```python
from build123d import *

# Parameters (mm, degrees)
SKETCH1_W           = 282
SKETCH1_H           = 170
BOSS_EXTRUDE1_DEPTH = 60
CUT_EXTRUDE4_DEPTH  = 5
SKETCH8_W           = 160
SKETCH8_H           = 50
CUT_EXTRUDE5_DEPTH  = 279
CUT_EXTRUDE6_DEPTH  = 5
SKETCH10_R          = 5
CUT_EXTRUDE7_DEPTH  = 5
CUT_EXTRUDE8_DEPTH  = 5
CUT_EXTRUDE9_START  = -5
CUT_EXTRUDE9_DEPTH  = 5
SKETCH14_W          = 185
SKETCH14_H          = 5
BOSS_EXTRUDE2_DEPTH = 10
SKETCH15_W          = 185
SKETCH15_H          = 5
BOSS_EXTRUDE3_DEPTH = 10
SKETCH16_W          = 97
SKETCH16_H          = 15
CUT_EXTRUDE10_DEPTH = 170
BOSS_EXTRUDE4_DEPTH = 160
SKETCH18_W          = 15
SKETCH18_H          = 10
CUT_EXTRUDE11_DEPTH = 340.888216918


with BuildPart() as part:
    # Sketch1 → Boss-Extrude1 (new body)
    with BuildSketch(Plane(origin=(0, 0, 0), x_dir=(1, 0, 0), z_dir=(0, 1, 0))):
        with Locations((141, 85)):
            Rectangle(SKETCH1_W, SKETCH1_H)
    extrude(amount=BOSS_EXTRUDE1_DEPTH)

    # Sketch7 → Cut-Extrude4 (cut)
    with BuildSketch(Plane.XZ):
        with BuildLine():
            Line((13.5, -37.5), (13.5, -132.5))
            ThreePointArc((13.5, -132.5), (11, -135), (8.5, -132.5))
            Line((8.5, -132.5), (8.5, -37.5))
            ThreePointArc((8.5, -37.5), (11, -35), (13.5, -37.5))
        make_face()
        with BuildLine():
            Line((58.5, -37.5), (58.5, -132.5))
            ThreePointArc((58.5, -132.5), (56, -135), (53.5, -132.5))
            Line((53.5, -132.5), (53.5, -37.5))
            ThreePointArc((53.5, -37.5), (56, -35), (58.5, -37.5))
        make_face()
        with BuildLine():
            Line((28.5, -37.5), (28.5, -132.5))
            ThreePointArc((28.5, -132.5), (26, -135), (23.5, -132.5))
            Line((23.5, -132.5), (23.5, -37.5))
            ThreePointArc((23.5, -37.5), (26, -35), (28.5, -37.5))
        make_face()
        with BuildLine():
            Line((43.5, -37.5), (43.5, -132.5))
            ThreePointArc((43.5, -132.5), (41, -135), (38.5, -132.5))
            Line((38.5, -132.5), (38.5, -37.5))
            ThreePointArc((38.5, -37.5), (41, -35), (43.5, -37.5))
        make_face()
    extrude(amount=-CUT_EXTRUDE4_DEPTH, mode=Mode.SUBTRACT)

    # Sketch8 → Cut-Extrude5 (cut)
    with BuildSketch(Plane(origin=(282, 0, 0), x_dir=(0, 0, -1), z_dir=(1, 0, 0))):
        with Locations((85, 30)):
            Rectangle(SKETCH8_W, SKETCH8_H)
    extrude(amount=-CUT_EXTRUDE5_DEPTH, mode=Mode.SUBTRACT)

    # Sketch9 → Cut-Extrude6 (cut)
    with BuildSketch(Plane.XY):
        Polygon((217.15, 25.8), (227.05, 25.8), (227.05, 8.15), (224.8, 5), (219.4, 5), (217.15, 8.15), align=None)
        Polygon((162.25, 25.8), (172.15, 25.8), (172.15, 8.15), (169.9, 5), (164.5, 5), (162.25, 8.15), align=None)
    extrude(amount=-CUT_EXTRUDE6_DEPTH, mode=Mode.SUBTRACT)

    # Sketch10 → Cut-Extrude7 (cut)
    with BuildSketch(Plane.ZY):
        with Locations((-129.202249563, 20)):
            Circle(SKETCH10_R)
        with Locations((-114.202249563, 20)):
            Circle(SKETCH10_R)
        with Locations((-99.202249563, 20)):
            Circle(SKETCH10_R)
        with Locations((-43.390057257, 20)):
            Circle(SKETCH10_R)
        with Locations((-58.390057257, 20)):
            Circle(SKETCH10_R)
        with Locations((-73.390057257, 20)):
            Circle(SKETCH10_R)
    extrude(amount=-CUT_EXTRUDE7_DEPTH, mode=Mode.SUBTRACT)

    # Sketch11 → Cut-Extrude8 (cut)
    with BuildSketch(Plane.XY):
        with BuildLine():
            Line((11, 13.5), (56, 13.5))
            ThreePointArc((56, 13.5), (58.5, 11), (56, 8.5))
            Line((56, 8.5), (11, 8.5))
            ThreePointArc((11, 8.5), (8.5, 11), (11, 13.5))
        make_face()
        with BuildLine():
            Line((11, 23.5), (56, 23.5))
            ThreePointArc((56, 23.5), (58.5, 21), (56, 18.5))
            Line((56, 18.5), (11, 18.5))
            ThreePointArc((11, 18.5), (8.5, 21), (11, 23.5))
        make_face()
    extrude(amount=-CUT_EXTRUDE8_DEPTH, mode=Mode.SUBTRACT)

    # Sketch12 → Cut-Extrude9 (cut)
    with BuildSketch(Plane(origin=(0, 0, -170), x_dir=(-1, 0, 0), z_dir=(0, 0, -1)).offset(CUT_EXTRUDE9_START)):
        with BuildLine():
            Line((-56, 13.5), (-11, 13.5))
            ThreePointArc((-11, 13.5), (-8.5, 11), (-11, 8.5))
            Line((-11, 8.5), (-56, 8.5))
            ThreePointArc((-56, 8.5), (-58.5, 11), (-56, 13.5))
        make_face()
        with BuildLine():
            Line((-56, 23.5), (-11, 23.5))
            ThreePointArc((-11, 23.5), (-8.5, 21), (-11, 18.5))
            Line((-11, 18.5), (-56, 18.5))
            ThreePointArc((-56, 18.5), (-58.5, 21), (-56, 23.5))
        make_face()
    extrude(amount=CUT_EXTRUDE9_DEPTH, mode=Mode.SUBTRACT)

    # Sketch14 → Boss-Extrude2 (add)
    with BuildSketch(Plane.XY):
        with Locations((189.5, 57.5)):
            Rectangle(SKETCH14_W, SKETCH14_H)
    extrude(amount=BOSS_EXTRUDE2_DEPTH)

    # Sketch15 → Boss-Extrude3 (add)
    with BuildSketch(Plane(origin=(0, 0, -170), x_dir=(-1, 0, 0), z_dir=(0, 0, -1))):
        with Locations((-189.5, 57.5)):
            Rectangle(SKETCH15_W, SKETCH15_H)
    extrude(amount=BOSS_EXTRUDE3_DEPTH)

    # Sketch16 → Cut-Extrude10 (cut)
    with BuildSketch(Plane.XY):
        with Locations((48.5, 52.5)):
            Rectangle(SKETCH16_W, SKETCH16_H)
    extrude(amount=-CUT_EXTRUDE10_DEPTH, mode=Mode.SUBTRACT)

    # Sketch17 → Boss-Extrude4 (add)
    with BuildSketch(Plane.XY.offset(-165)):
        Polygon((3, 45), (97, 45), (97, 55), (102, 55), (102, 40), (3, 40), align=None)
    extrude(amount=BOSS_EXTRUDE4_DEPTH)

    # Sketch18 → Cut-Extrude11 (cut, through all)
    with BuildSketch(Plane.XY):
        with Locations((69.5, 22)):
            Rectangle(SKETCH18_W, SKETCH18_H)
    extrude(amount=-CUT_EXTRUDE11_DEPTH, mode=Mode.SUBTRACT)


solid = part.part
```
The listing builds one solid part. Answer for the finished solid, in the listing's coordinates (mm). A direction names the side the tool comes from. Give positions to 0.01 mm unless a question says otherwise; leave off trailing zeros. Order: outer loops, then holes, each group sorted by start corner. A loop starts at its lowest first (then second) coordinate and runs counter-clockwise, first axis right, second up.
1) Given P1, Ø5, axis at x = 147, y = 50.5, coming from the -Z side; P2, Ø8, axis at y = 9.5, z = -30, coming from the -X side; P3, Ø5, axis at y = 11.5, z = -103.5, coming from the +X side; P4, Ø12, axis at y = 48.5, z = -74, coming from the +X side, each flat-ended and moving along its own axis, determine where each tip first touches the part or whether it passes through.
Reported:
P1: stops at z = -170
P2: stops at x = 0
P3: stops at x = 3
P4: stops at x = 102
2) For faces 5 (the face through (191, 55, -175)), 6 (the face through (97, 52, -86)), 7 (the face through (175, 30, -5)), determine the directions among +Z, -Z, +X, -X, +Y, -Y from which every point of the face is accessible in a straight line to the end or side of a thin tool.
Reported:
face 5: -Z, +X, -X, -Y
face 6: +Z, -Z, -X, +Y
face 7: +X
3) Find section A-A on x = 18. Write down the section's boundary in (y, z), then the cut area to 3 significant figures.
Reported:
outline: (0, -170) - (8.5, -170) - (8.5, -165) - (5, -165) - (5, -5) - (8.5, -5) - (8.5, 0) - (0, 0) - close; (13.5, -170) - (18.5, -170) - (18.5, -165) - (13.5, -165) - close; (13.5, -5) - (18.5, -5) - (18.5, 0) - (13.5, 0) - close; (23.5, -170) - (45, -170) - (45, 0) - (23.5, 0) - (23.5, -5) - (40, -5) - (40, -165) - (23.5, -165) - close
area: 1,950 mm2
4) Find section C-C on x = 130.5. Write down the section's boundary in (y, z).
Reported:
outline: (0, -170) - (55, -170) - (55, -180) - (60, -180) - (60, 10) - (55, 10) - (55, 0) - (0, 0) - close; hole (5, -165) - (55, -165) - (55, -5) - (5, -5) - close
5) Consider line 1 along Y through (x, z) = (58, -163); line 2 along Y through (x, z) = (238, -44); line 3 along Z through (x, y) = (63.5, 28). Determine where each line is inside the solid, lowest interval first.
Reported:
line 1: y = 0 to 5, 40 to 45
line 2: y = 0 to 5, 55 to 60
line 3: z = -170 to -165, -5 to 0
6) Determine the mould class of faces 1 (the face through (48, 45, -86)), 2 (the face through (139, 27, -170)), 3 (the face through (1.479, 15.564, -41.083)), 4 (the face through (3, 23, -84)) for opening direction Z: pulls with the +Z half, pulls with the -Z half, needs draft (parallel to the pull), parting line crosses it, or undercut.
Reported:
face 1: needs draft
face 2: pulls with the -Z half
face 3: undercut
face 4: undercut
7) Find section D-D on y = 33. Write down the section's boundary in (x, z).
Reported:
outline: (0, -170) - (282, -170) - (282, -165) - (3, -165) - (3, -5) - (282, -5) - (282, 0) - (0, 0) - close
8) Find section B-B on z = -157. Write down the section's boundary in (x, y), then the cut area to 3 significant figures.
Reported:
outline: (0, 0) - (282, 0) - (282, 5) - (3, 5) - (3, 40) - (102, 40) - (102, 55) - (282, 55) - (282, 60) - (97, 60) - (97, 45) - (0, 45) - close
area: 3,000 mm2
